Input: part model. Units: mm. Frame: model coordinates. Face numbers are marked on the shaded views. Give positions to 0.01 mm unless a question says otherwise; leave off trailing zeros. Loops run counter-clockwise (first coordinate to the right, second up) from the corner with the lowest first, then second, coordinate; pieces in that order, holes last. Notation, with made-up numbers: M -7,51 L 50,51 A22 cw 50,74 Z; hole C 80,53 d9. An arc over 180 degrees is marked long. Answer as a JSON object with one key per item and string values. Group by question number.
1) Section query D-D on x = 14. Return loops of the section in (y, z).
2) Section query C-C on x = 141. Return loops of the section in (y, z).
3) Section query A-A on y = -10. Return loops of the section in (x, z), plus the area to 3 significant figures.
4) Ray query, L1, parallel to X at y = -7.75, z = 28.5; L2, parallel to Y at x = 12, z = 6; L3, parallel to X at y = -1.25, z = -50. Return the intervals inside material, ascending.
5) Section query B-B on z = 18. Return loops of the section in (x, y).
6) First-contact query: P1, Ø5.5, axis at y = -9.5, z = -48, coming from the +X side; P2, Ø3, axis at x = -3.5, y = -4.5, coming from the +Z side; P3, Ø5.5, axis at x = -2.5, y = -9.5, coming from the +Z side. Flat tips, straight axial feed; report the tip coordinate or a pass-through.
7) Draft query along X for the marked faces 1, 2 and 3. Return one class per face: +X half, -X half, draft (parallel to the pull), parting line (faces both ways), or undercut.
from build123d import *

# Parameters (mm, degrees)
SKETCH1_W           = 342.9
SKETCH1_H           = 127
BOSS_EXTRUDE1_DEPTH = 12.7
DRAFT1_ANGLE        = -45
SKETCH2_W           = 23.368
SKETCH2_H           = 127
CUT_EXTRUDE1_DEPTH  = 5.08
CUT_EXTRUDE2_DEPTH  = 5.08
SKETCH4_W           = 81.661
SKETCH4_H           = 26.162
CUT_EXTRUDE3_DEPTH  = 5.08
SKETCH5_W           = 72.464825645
SKETCH5_H           = 13.081
CUT_EXTRUDE4_DEPTH  = 184.272045059
FILLET1_R           = 6.604


with BuildPart() as part:
    # Sketch1 → Boss-Extrude1 (new body)
    with BuildSketch(Plane(origin=(0, 0, 0), x_dir=(1, 0, 0), z_dir=(0, 1, 0))):
        Rectangle(SKETCH1_W, SKETCH1_H)
    extrude(amount=-BOSS_EXTRUDE1_DEPTH)

    # Draft1
    draft1_faces = [part.faces().sort_by_distance(p)[0] for p in [
        (0, -6.35, -63.5),
        (-171.45, -6.35, 0),
        (171.45, -6.35, 0),
        (0, -6.35, 63.5),
    ]]
    draft(draft1_faces, Plane.ZX, DRAFT1_ANGLE)

    # Sketch2 → Cut-Extrude1 (cut)
    with BuildSketch(Plane.XZ.offset(12.7)):
        with Locations((12.446, 0)):
            Rectangle(SKETCH2_W, SKETCH2_H)
    extrude(amount=-CUT_EXTRUDE1_DEPTH, mode=Mode.SUBTRACT)

    # Sketch3 → Cut-Extrude2 (cut)
    with BuildSketch(Plane.XZ.offset(12.7)):
        with BuildLine():
            Line((0.762, 55.88), (-19.431, 55.88))
            Line((-19.431, 55.88), (-19.431, 30.988))
            ThreePointArc((-19.431, 30.988), (-12.827, 24.384), (-6.223, 30.988))
            Line((-6.223, 30.988), (0.762, 30.988))
            Line((0.762, 30.988), (0.762, 55.88))
        make_face()
    extrude(amount=-CUT_EXTRUDE2_DEPTH, mode=Mode.SUBTRACT)

    # Sketch4 → Cut-Extrude3 (cut)
    with BuildSketch(Plane.XZ.offset(12.7)):
        with Locations((130.6195, -50.419)):
            Rectangle(SKETCH4_W, SKETCH4_H)
    extrude(amount=-CUT_EXTRUDE3_DEPTH, mode=Mode.SUBTRACT)

    # Sketch5 → Cut-Extrude4 (cut, through all)
    with BuildSketch(Plane.XZ.offset(12.7)):
        with Locations((135.217587178, -56.9595)):
            Rectangle(SKETCH5_W, SKETCH5_H)
    extrude(amount=-CUT_EXTRUDE4_DEPTH, mode=Mode.SUBTRACT)

    # Fillet1
    fillet1_edges = [part.edges().sort_by_distance(p)[0] for p in [
        (98.985174355, -3.81, -50.419),
    ]]
    fillet(fillet1_edges, radius=FILLET1_R)


solid = part.part
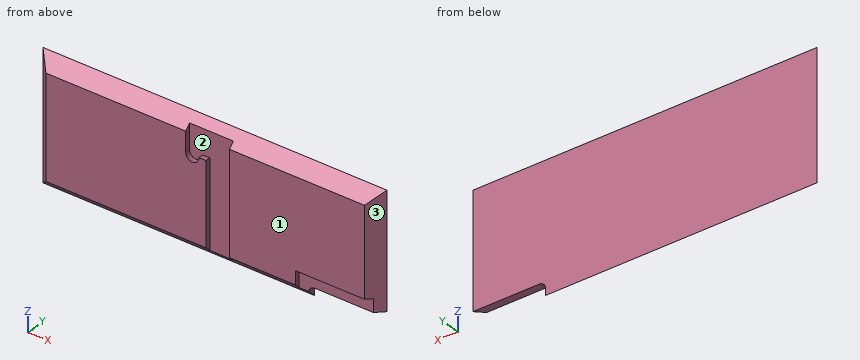
Output:
{
 "1": {"outline": "M -7.62,-55.88 L 0,-63.5 L 0,63.5 L -7.62,55.88 Z"},
 "2": {"outline": "M -12.7,-37.34 L -7.62,-37.34 L -7.62,-50.42 L 0,-50.42 L 0,63.5 L -12.7,50.8 Z"},
 "3": {"outline": "M -161.45,-53.5 L 0.76,-53.5 L 0.76,30.99 L -6.22,30.99 A6.6 cw -19.43,30.99 L -19.43,53.5 L -161.45,53.5 Z; M 24.13,-53.5 L 89.79,-53.5 L 89.79,-37.34 L 161.45,-37.34 L 161.45,53.5 L 24.13,53.5 Z", "area": "30,400 mm^2"},
 "4": {"L1": "x = -163.7 to -18.94, -6.71 to 0.76, 24.13 to 163.7", "L2": "y = -7.62 to 0", "L3": "x = -170.2 to 170.2"},
 "5": {"outline": "M -171.45,0 L -158.75,-12.7 L 0.76,-12.7 L 0.76,-7.62 L 24.13,-7.62 L 24.13,-12.7 L 158.75,-12.7 L 171.45,0 Z"},
 "6": {"P1": "stops at x = 164.7", "P2": "stops at z = 60.5", "P3": "stops at z = 56.75"},
 "7": {"face 1": "draft", "face 2": "undercut", "face 3": "+X half"}
}
